The model under review builds one solid part; all positions refer to its coordinate system, in mm. Face numbers are marked on the shaded views. A direction names the side the tool comes from. Coordinates: 2 decimals unless noted, no trailing zeros. Write each loop counter-clockwise with the first axis right and the second up, starting at its lowest first coordinate (ties: lowest second). Pieces come first, ordered by that corner, then holes.
1) Add section D-D, the plane x = -0.5. State the section outline as (y, z) points, then the cut area to 3 significant figures.
2) For P1, Ø1, axis at x = 2.5, z = -0.5, coming from the +Y side; P2, Ø1.5, axis at x = -1.5, z = 1, coming from the -Y side, all flat-tipped, find the tip position at first contact; note any pin that passes through.
3) Add section C-C, the plane x = 1. State the section outline as (y, z) points, then the cut area to 3 significant figures.
4) For line 1 (X direction, y = 0.2, z = -1.45) (3 decimals); line 2 (Y direction, x = 4.5, z = 0.05); line 3 (Z direction, x = -2.25, y = 0.9), list the stretches that pass through material, from the lowest coordinate up.
5) Machinability: for the marked faces 1 and 2, which of the approach directions +Z, -Z, +X, -X, +Y, -Y give a long, thin tool a straight path to every point of the face, cutting with its end or side? Answer none if there is none.
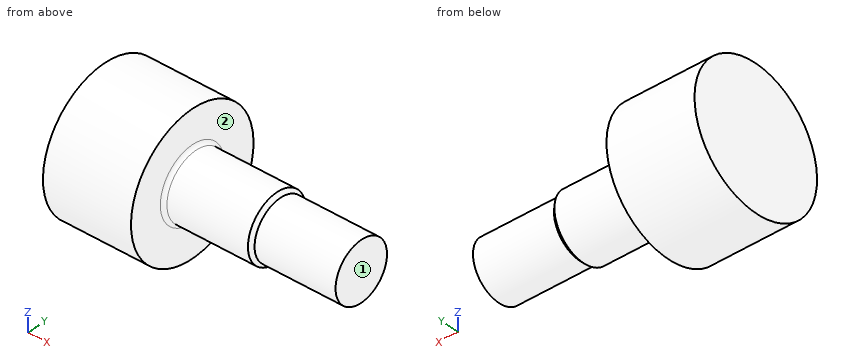
from build123d import *

# Parameters (mm, degrees)
F0_W     = 2.921
F0_H     = 1.05664
F2_R     = 0.127
F3_SIZE2 = 0.12699
F3_SIZE  = 0.12699


# Not quite as in the source:
# - a fillet or chamfer is up to 0.001 mm smaller than in the source, because OpenCascade refuses the exact size


with BuildPart() as f1:
    # F0 (on Front) → F1 (revolve)
    with BuildSketch(Plane.XZ):
        Polygon((-3.175, 0), (0, 0), (0, 1.18364), (0, 2.5146), (-3.175, 2.5146), align=None)
        Polygon((0, 1.18364), (0, 0), (3.175, 0), (3.175, 1.05664), (3.175, 1.18364), align=None)
        with Locations((4.6355, 0.52832)):
            Rectangle(F0_W, F0_H)
    revolve(axis=Axis((-1.5875, 0, 0), (-1, 0, 0)))

    # F2
    f2_edges = [f1.edges().sort_by_distance(p)[0] for p in [
        (0, 0, -1.18364),
    ]]
    fillet(f2_edges, radius=F2_R)

    # F3 (size 0.127 and 0.127 in the source; OpenCascade refuses exactly that, so slightly less here)
    f3_edges = [f1.edges().sort_by_distance(p)[0] for p in [
        (3.175, 0, -1.18364),
    ]]
    chamfer(f3_edges, length=F3_SIZE, length2=F3_SIZE2)


solid = f1.part
Geometry results:
1. outline: circle Ø5.03 at (0, 0)
1. area: 19.9 mm2
2. P1: stops at y = 1.18
2. P2: stops at y = -2.5
3. outline: circle Ø2.37 at (0, 0)
3. area: 4.40 mm2
4. line 1: x = -3.175 to 0
4. line 2: y = -1.06 to 1.06
4. line 3: z = -2.35 to 2.35
5. face 1: +Z, -Z, +X, +Y, -Y
5. face 2: +X
